```python
from build123d import *

# Parameters (mm, degrees)
CHAMFER_1_SIZE      = 0.5
SKETCH_2_W          = 1
SKETCH_2_H          = 14.5
CUT_EXTRUDE_2_DEPTH = 4.5


with BuildPart() as part:
    # Эскиз1 → Повернуть1 (revolve)
    with BuildSketch(Plane.XY):
        Polygon((0, 7.95), (1.5, 7.95), (0, 10.548076211), (0, 14), (-2, 14), (-2, 8.485898385), align=None)
    revolve(axis=Axis((-6.176798117, 0, 0), (1, 0, 0)))

    # Фаска1
    chamfer_1_edges = [part.edges().sort_by_distance(p)[0] for p in [
        (0, -14, 0),
    ]]
    chamfer(chamfer_1_edges, length=CHAMFER_1_SIZE)

    # Эскиз2 → Вырез-Вытянуть2 (cut, through all)
    with BuildSketch(Plane.ZY.offset(2)):
        with Locations((0, 7.25)):
            Rectangle(SKETCH_2_W, SKETCH_2_H)
    extrude(amount=-CUT_EXTRUDE_2_DEPTH, mode=Mode.SUBTRACT)


solid = part.part
```
For this review, take the finished solid that the model builds, in its own axes (mm). A direction names the side the tool comes from. Coordinates: 2 decimals unless noted, no trailing zeros. Write each loop counter-clockwise with the first axis right and the second up, starting at its lowest first coordinate (ties: lowest second). Pieces come first, ordered by that corner, then holes. Notation, with made-up numbers: (5, -14) -> (33, -14) arc R10 ccw to (33, -8) -> close; hole circle Ø10 at (-26, 0). An arc over 180 degrees is marked (long way). Put each result on its own line as item: value.
Q1. Take a section at C-C, the plane x = 1.1. State the section outline as (y, z) points, then the cut area to 3 significant figures.
From the geometry:
outline: (7.93, -0.5) arc R7.95 cw (long way) to (7.93, 0.5) -> (8.63, 0.5) arc R8.64 ccw (long way) to (8.63, -0.5) -> close
area: 35.4 mm2
Q2. Tool access review of faces 1 (the flat face through (-1, 11, 0.5)), 2 (the cylindrical face through (-1.26, -13.987, 0.609)): name each direction out of +Z, -Z, +X, -X, +Y, -Y from which nothing blocks a thin tool from reaching the whole face with its end or side.
From the geometry:
face 1: +X, -X, +Y
face 2: +X, -X
Q3. Wall thickness on L1, parallel to X at y = 9.75, z = -9; L2, parallel to Y at x = 0.05, z = 1.75 (3 decimals); L3, parallel to Z at x = 0.5, y = 0: over which ranges is each line inside the solid? List them lowest first.
From the geometry:
L1: x = -2 to 0
L2: y = -10.314 to -7.755, 7.755 to 10.314
L3: z = -9.68 to -7.95, 7.95 to 9.68
Q4. The part is to be moulded in two halves that separate along Z. For faces 3 (the flat face through (0, -4, 10)), 4 (the conical face through (1.41, -8.1, 0.35)), 5 (the conical face through (-0.32, -8.03, 0.35)), say which applies: +Z half, -Z half, draft (parallel to the pull), parting line (faces both ways), or undercut.
From the geometry:
face 3: draft
face 4: parting line
face 5: undercut
Q5. Take a section at B-B, the plane z = 0. State the section outline as (x, y) points.
From the geometry:
outline: (-2, -14) -> (-0.5, -14) -> (0, -13.5) -> (0, -10.55) -> (1.5, -7.95) -> (0, -7.95) -> (-2, -8.49) -> close
Q6. Clearance check with flat-ended pins moving along their axes: pin 1 Ø1.5 at (x, z) = (-1, 10.5) entering from +Y; pin 2 Ø1.8 at (x, y) = (-0.5, 11) entering from -Z. State where each tip first meets the part, or that it passes through.
From the geometry:
pin 1: stops at y = 10.05
pin 2: stops at z = -9.69
Q7. Take a section at A-A, the plane y = 0. State the section outline as (x, z) points, then the cut area to 3 significant figures.
From the geometry:
outline: (-2, -14) -> (-0.5, -14) -> (0, -13.5) -> (0, -10.55) -> (1.5, -7.95) -> (0, -7.95) -> (-2, -8.49) -> close; (-2, 8.49) -> (0, 7.95) -> (1.5, 7.95) -> (0, 10.55) -> (0, 13.5) -> (-0.5, 14) -> (-2, 14) -> close
area: 26.8 mm2
